Geometry: final body of the model. Coordinates: model frame, mm. Face numbers are marked on the shaded views. Round coordinates to 2 decimals unless told otherwise and drop trailing zeros. Loops run counter-clockwise (first coordinate to the right, second up) from the corner with the lowest first, then second, coordinate; pieces in that order, holes last. Notation, with made-up numbers: (-0.75, 44) -> (54.25, 44) arc R27 ccw to (54.25, 71) -> close; hole circle Ø5 at (32.25, 27). An arc over 180 degrees is marked (long way). Answer in a Markdown table with one row per item.
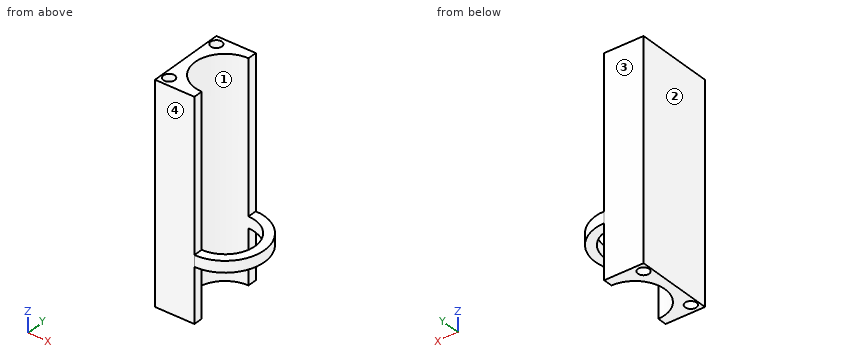
```python
from build123d import *

# Parameters (mm, degrees)
BOSS_EXTRUDE1_DEPTH       = 57.43
SKETCH2_W                 = 3
SKETCH2_H                 = 2.5
SKETCH6_R                 = 1.5
CUT_EXTRUDE1_DEPTH        = 0.1
CUT_EXTRUDE2_START        = -0.1
SKETCH9_R                 = 1.5
CUT_EXTRUDE2_DEPTH        = 0.1
F_3_0MM_DOWEL_HOLE1_D     = 3
F_3_0MM_DOWEL_HOLE1_DEPTH = 3
F_3_0MM_DOWEL_HOLE1_TIP   = 0.901290929
F_3_0MM_DOWEL_HOLE2_D     = 3
F_3_0MM_DOWEL_HOLE2_DEPTH = 3
F_3_0MM_DOWEL_HOLE2_TIP   = 0.901290929


with BuildPart() as part:
    # Sketch1 → Boss-Extrude1 (new body)
    with BuildSketch(Plane.XY):
        with BuildLine():
            Line((0, -8), (0, -10.5))
            Line((0, -10.5), (-10.5, -10.5))
            Line((-10.5, -10.5), (-10.5, 10.5))
            Line((-10.5, 10.5), (0, 10.5))
            Line((0, 10.5), (0, 8))
            ThreePointArc((0, 8), (-8, 0), (0, -8))
        make_face()
    extrude(amount=BOSS_EXTRUDE1_DEPTH)

    # Sketch2 → Revolve1 (revolve)
    with BuildSketch(Plane(origin=(0, 0, 0), x_dir=(0, 0, -1), z_dir=(1, 0, 0)), mode=Mode.PRIVATE) as revolve1_sk:
        with Locations((-15.93, -9.25)):
            Rectangle(SKETCH2_W, SKETCH2_H)
    revolve(revolve1_sk.sketch.rotate(Axis((0, 0, 0), (0, 0, 1)), 180), axis=Axis((0, 0, 0), (0, 0, 1)))

    # Sketch6 → Cut-Extrude1 (cut)
    with BuildSketch(Plane.XY.offset(57.43)):
        with Locations((-8.613344298, 8.08)):
            Circle(SKETCH6_R)
        with Locations((-8.613344298, -8.08)):
            Circle(SKETCH6_R)
    extrude(amount=-CUT_EXTRUDE1_DEPTH, mode=Mode.SUBTRACT)

    # Sketch9 → Cut-Extrude2 (cut)
    with BuildSketch(Plane(origin=(0, 0, 0), x_dir=(-1, 0, 0), z_dir=(0, 0, -1)).offset(CUT_EXTRUDE2_START)):
        with Locations(Location((8.613344298, 8.08, 0), (0, 0, 180))):
            Circle(SKETCH9_R)
        with Locations(Location((8.613344298, -8.08, 0), (0, 0, 180))):
            Circle(SKETCH9_R)
    extrude(amount=CUT_EXTRUDE2_DEPTH, mode=Mode.SUBTRACT)

    # Ø3.0mm Dowel Hole1
    with Locations(Plane.XY.offset(57.43)):
        with Locations((-8.613344298, 8.08), (-8.613344298, -8.08)):
            Hole(F_3_0MM_DOWEL_HOLE1_D / 2, depth=F_3_0MM_DOWEL_HOLE1_DEPTH)
            with Locations((0, 0, -(F_3_0MM_DOWEL_HOLE1_DEPTH + F_3_0MM_DOWEL_HOLE1_TIP / 2))):  # 118° drill point
                Cone(0, F_3_0MM_DOWEL_HOLE1_D / 2, F_3_0MM_DOWEL_HOLE1_TIP, mode=Mode.SUBTRACT)

    # Ø3.0mm Dowel Hole2
    with Locations(Plane(origin=(0, 0, 0), x_dir=(-1, 0, 0), z_dir=(0, 0, -1))):
        with Locations((8.613344298, 8.08), (8.613344298, -8.08)):
            Hole(F_3_0MM_DOWEL_HOLE2_D / 2, depth=F_3_0MM_DOWEL_HOLE2_DEPTH)
            with Locations((0, 0, -(F_3_0MM_DOWEL_HOLE2_DEPTH + F_3_0MM_DOWEL_HOLE2_TIP / 2))):  # 118° drill point
                Cone(0, F_3_0MM_DOWEL_HOLE2_D / 2, F_3_0MM_DOWEL_HOLE2_TIP, mode=Mode.SUBTRACT)


solid = part.part
```
Item 1: Section query A-A, the plane y = 0. Output: boundary loops of the cut face in (x, z), and give its area (3 significant figures).
Ans:
| item | result |
|---|---|
| outline | (-10.5, 0) -> (-8, 0) -> (-8, 57.43) -> (-10.5, 57.43) -> close; (8, 14.43) -> (10.5, 14.43) -> (10.5, 17.43) -> (8, 17.43) -> close |
| area | 151 mm2 |
Item 2: First-contact query: P1, Ø2.5, axis at x = -8.61, y = 8.08, coming from the -Z side; P2, Ø1.2, axis at y = 9, z = 42.5, coming from the +X side; P3, Ø3, axis at x = 7.5, y = 4, coming from the +Z side. Flat tips, straight axial feed; report the tip coordinate or a pass-through.
Ans:
| item | result |
|---|---|
| P1 | z = 3.15 |
| P2 | x = 0 |
| P3 | z = 17.43 |
Item 3: Ray query, L1, parallel to X at y = 8.08, z = 55.75; L2, parallel to X at y = 0, z = 22.5; L3, parallel to Y at x = -1.5, z = 25. Return the intervals inside material, ascending.
Ans:
| item | result |
|---|---|
| L1 | -10.5 to -10.11, -7.11 to 0 |
| L2 | -10.5 to -8 |
| L3 | -10.5 to -7.86, 7.86 to 10.5 |
Item 4: Section query B-B, the plane z = 27. Output: boundary loops of the cut face in (x, y).
Ans:
| item | result |
|---|---|
| outline | (-10.5, -10.5) -> (0, -10.5) -> (0, -8) arc R8 cw to (0, 8) -> (0, 10.5) -> (-10.5, 10.5) -> close |
Item 5: Mould query, pull axis Y, two halves, no side actions, for the marked faces 1, 2, 3 and 4. Classes: released by +Y, released by -Y, zero draft, split by the parting line, or undercut.
Ans:
| item | result |
|---|---|
| face 1 | undercut |
| face 2 | zero draft |
| face 3 | released by +Y |
| face 4 | released by -Y |
Item 6: Section query C-C, the plane x = -6. Output: boundary loops of the cut face in (y, z).
Ans:
| item | result |
|---|---|
| outline | (-10.5, 0) -> (-5.29, 0) -> (-5.29, 57.43) -> (-10.5, 57.43) -> close; (5.29, 0) -> (10.5, 0) -> (10.5, 57.43) -> (5.29, 57.43) -> close |
